The figure shows three views and two pictorial views of one solid part (mm, origin at its lowest corner). Answer the questions. Coordinates: 2 decimals unless noted, no trailing zeros. Order: outer loops, then holes, each group sorted by start corner. A loop starts at its lowest first (then second) coordinate and runs counter-clockwise, first axis right, second up.
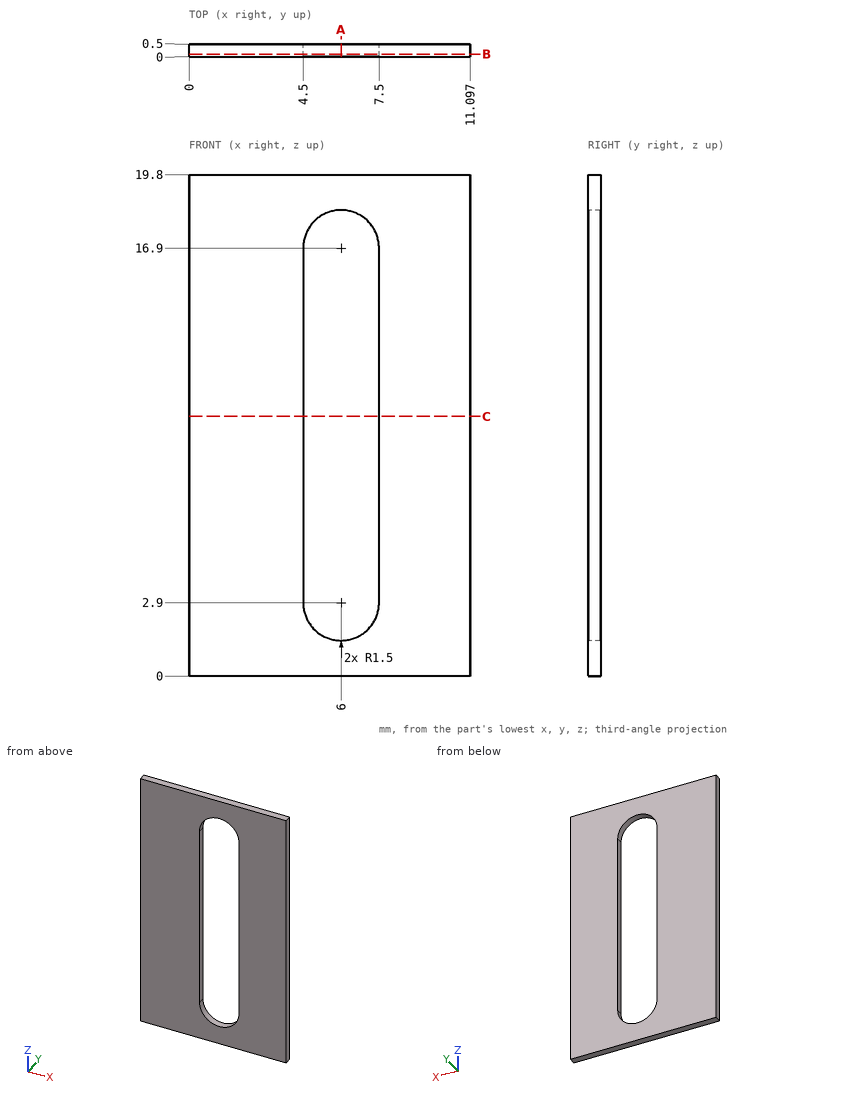
Q1. The part is cut by section B-B, the plane y = 0.1. Determine the outline of the cut face in (x, z).
Q2. Straight lines are drawn through the part: L1, parallel to X at y = 0.35, z = 16.25; L2, parallel to Z at x = 6.5, y = 0.05; L3, parallel to X at y = 0.1, z = 2.5. For each, find the intervals that lie inside material, in ascending order.
Q3. The part is cut by section A-A, the plane x = 6. Determine the outline of the cut face in (y, z).
Q4. The part is cut by section C-C, the plane z = 10.25. Determine the outline of the cut face in (x, y).
Computed values:
1. outline: (0, 0) - (11.1, 0) - (11.1, 19.8) - (0, 19.8) - close; hole (4.5, 2.9) arc R1.5 ccw to (7.5, 2.9) - (7.5, 16.9) arc R1.5 ccw to (4.5, 16.9) - close
2. L1: x = 0 to 4.5, 7.5 to 11.1
2. L2: z = 0 to 1.49, 18.31 to 19.8
2. L3: x = 0 to 4.55, 7.45 to 11.1
3. outline: (0, 0) - (0.5, 0) - (0.5, 1.4) - (0, 1.4) - close; (0, 18.4) - (0.5, 18.4) - (0.5, 19.8) - (0, 19.8) - close
4. outline: (0, 0) - (4.5, 0) - (4.5, 0.5) - (0, 0.5) - close; (7.5, 0) - (11.1, 0) - (11.1, 0.5) - (7.5, 0.5) - close
